Build history of the part. All positions in model axes, mm. Round coordinates to 2 decimals unless told otherwise and drop trailing zeros. Answer as a JSON object with one key per item and string values. Group by question number.
Item 1: Slice it at A-A, the plane y = -69.5. Give the number of separate pieces and of enclosed holes in the cut face, then the cut area to 3 significant figures.
Item 2: Flat gauge pins, fed straight in: pin 1 (7 mm diameter, centred on x = 9.5, y = -33, fed in from -Z); pin 2 (5 mm diameter, centred on x = 31, y = -45.5, fed in from +Z); pin 3 (3 mm diameter, centred on x = -4, y = -32.5, fed in from -Z). Where does each tip first touch, or does it go through?
Item 3: Probe line 1 (X direction, y = -24.5, z = -15); line 2 (X direction, y = -17.5, z = 12.5); line 3 (Z direction, x = -17, y = -14.5). List the from-to ranges inside material, lowest first. Write a range as from..to.
from build123d import *

# Parameters (mm, degrees)
F0_R     = 47.625
F1_DEPTH = 76.2
F3_DEPTH = 76.201


with BuildPart() as f1:
    # F0 (on Front) → F1 (new body)
    with BuildSketch(Plane.XZ):
        Circle(F0_R)
    extrude(amount=F1_DEPTH)

    # F2 (on face) → F3 (cut, through all)
    with BuildSketch(Plane.XZ.offset(76.2)):
        Polygon((-16.073533, 25.021508), (-19.248533, 30.52077), (-25.598533, 30.52077), (-28.773533, 25.021508), (-25.598533, 19.522247), (-19.248533, 19.522247), align=None)
        Polygon((-0.733869, 35.056195), (-3.908869, 40.555456), (-10.258869, 40.555456), (-13.433869, 35.056195), (-10.258869, 29.556934), (-3.908869, 29.556934), align=None)
        Polygon((16.633373, 35.590573), (13.458373, 41.089834), (7.108373, 41.089834), (3.933373, 35.590573), (7.108373, 30.091312), (13.458373, 30.091312), align=None)
        Polygon((1.537231, 19.692863), (-1.637769, 25.192124), (-7.987769, 25.192124), (-11.162769, 19.692863), (-7.987769, 14.193602), (-1.637769, 14.193602), align=None)
        Polygon((16.633373, 21.295993), (13.458373, 26.795255), (7.108373, 26.795255), (3.933373, 21.295993), (7.108373, 15.796732), (13.458373, 15.796732), align=None)
        Polygon((30.393575, 26.372573), (27.218575, 31.871834), (20.868575, 31.871834), (17.693575, 26.372573), (20.868575, 20.873312), (27.218575, 20.873312), align=None)
        Polygon((37.073285, 12.077994), (33.898285, 17.577256), (27.548285, 17.577256), (24.373285, 12.077994), (27.548285, 6.578733), (33.898285, 6.578733), align=None)
        Polygon((17.969316, 6.467039), (14.794316, 11.9663), (8.444316, 11.9663), (5.269316, 6.467039), (8.444316, 0.967778), (14.794316, 0.967778), align=None)
        Polygon((-0.466681, 6.467039), (-3.641681, 11.9663), (-9.991681, 11.9663), (-13.166681, 6.467039), (-9.991681, 0.967778), (-3.641681, 0.967778), align=None)
        Polygon((-18.902677, 10.474864), (-22.077677, 15.974126), (-28.427677, 15.974126), (-31.602677, 10.474864), (-28.427677, 4.975603), (-22.077677, 4.975603), align=None)
        Polygon((-30.391778, 0.455301), (-33.566778, 5.954563), (-39.916778, 5.954563), (-43.091778, 0.455301), (-39.916778, -5.04396), (-33.566778, -5.04396), align=None)
        Polygon((-26.65114, -13.972871), (-29.82614, -8.47361), (-36.17614, -8.47361), (-39.35114, -13.972871), (-36.17614, -19.472132), (-29.82614, -19.472132), align=None)
        Polygon((-13.692505, -4.487684), (-16.867505, 1.011578), (-23.217505, 1.011578), (-26.392505, -4.487684), (-23.217505, -9.986945), (-16.867505, -9.986945), align=None)
        Polygon((1.670825, -7.56035), (-1.504175, -2.061088), (-7.854175, -2.061088), (-11.029175, -7.56035), (-7.854175, -13.059611), (-1.504175, -13.059611), align=None)
        Polygon((16.098997, -7.159568), (12.923997, -1.660306), (6.573997, -1.660306), (3.398997, -7.159568), (6.573997, -12.658829), (12.923997, -12.658829), align=None)
        Polygon((30.794357, -0.21267), (27.619357, 5.286592), (21.269357, 5.286592), (18.094357, -0.21267), (21.269357, -5.711931), (27.619357, -5.711931), align=None)
        Polygon((43.35221, -8.762698), (40.17721, -3.263437), (33.82721, -3.263437), (30.65221, -8.762698), (33.82721, -14.261959), (40.17721, -14.261959), align=None)
        Polygon((28.122474, -15.308812), (24.947474, -9.809551), (18.597474, -9.809551), (15.422474, -15.308812), (18.597474, -20.808074), (24.947474, -20.808074), align=None)
        Polygon((-12.688582, -19.25737), (-15.863582, -13.758108), (-22.213582, -13.758108), (-25.388582, -19.25737), (-22.213582, -24.756631), (-15.863582, -24.756631), align=None)
        Polygon((1.338806, -21.394878), (-1.836194, -15.895617), (-8.186194, -15.895617), (-11.361194, -21.394878), (-8.186194, -26.894139), (-1.836194, -26.894139), align=None)
        Polygon((15.900572, -23.933166), (12.725572, -18.433905), (6.375572, -18.433905), (3.200572, -23.933166), (6.375572, -29.432427), (12.725572, -29.432427), align=None)
        Polygon((0.865366, -34.677781), (-2.309634, -29.17852), (-8.659634, -29.17852), (-11.834634, -34.677781), (-8.659634, -40.177042), (-2.309634, -40.177042), align=None)
        Polygon((-14.291712, -33.551947), (-17.466712, -28.052686), (-23.816712, -28.052686), (-26.991712, -33.551947), (-23.816712, -39.051209), (-17.466712, -39.051209), align=None)
        Polygon((27.523267, -31.013658), (24.348267, -25.514396), (17.998267, -25.514396), (14.823267, -31.013658), (17.998267, -36.512919), (24.348267, -36.512919), align=None)
        Polygon((16.034166, -37.025397), (12.859166, -31.526136), (6.509166, -31.526136), (3.334166, -37.025397), (6.509166, -42.524658), (12.859166, -42.524658), align=None)
    extrude(amount=-F3_DEPTH, mode=Mode.SUBTRACT)


solid = f1.part
Geometry says:
{
 "1": {"separate pieces": "1", "enclosed holes": "25", "area": "4,510 mm^2"},
 "2": {"pin 1": "stops at z = -47.25", "pin 2": "stops at z = 38.16", "pin 3": "stops at z = -47.56"},
 "3": {"line 1": "x = -45.2..-38.76, -27.24..-22.93, -15.15..15.6, 27.94..45.2", "line 2": "x = -45.96..-30.43, -20.07..24.62, 36.83..45.96", "line 3": "z = -44.49..-38.24, -28.86..-24.76, -13.76..-9.99, 1.01..23.42, 26.63..44.49"}
}
